Read the model definition and answer for the solid it produces. Units are mm, in the model's axes. Face numbers are marked on the shaded views. A direction names the side the tool comes from. Coordinates: 2 decimals unless noted, no trailing zeros. Order: outer loops, then holes, each group sorted by start corner. A loop starts at its lowest first (then second) coordinate and runs counter-clockwise, first axis right, second up. Notation, with made-up numbers: (-8, 61.5) -> (48, 61.5) arc R10 ccw to (48, 78.5) -> close; hole circle Ø4 at (75, 36.5). An arc over 180 degrees is marked (long way). Answer as a JSON object with one key per item and string values. Group by question number.
1) Section B-B on x = 12 is taken. Determine the outline of the cut face in (y, z), and give its area (3 significant figures).
2) Section D-D on x = -21 is taken. Determine the outline of the cut face in (y, z), and give its area (3 significant figures).
3) A tool of negligible diameter and unlimited length cuts with its end or side. For the marked faces 1, 2 and 3, from which of +Z, -Z, +X, -X, +Y, -Y can it reach the whole face along a straight path? Write none if from no direction.
4) Determine the mould class of the marked faces 4, 5 and 6 for opening direction Z: released by +Z, released by -Z, zero draft, split by the parting line, or undercut.
5) Consider L1, parallel to Z at x = -8.5, y = 28; L2, parallel to Z at x = -13.5, y = 20.5; L3, parallel to X at y = 20.5, z = 13. Determine where each line is inside the solid, lowest interval first.
6) Section A-A on y = 16.5 is taken. Determine the outline of the cut face in (x, z).
7) Given pin 1 (8 mm diameter, centred on x = 3, y = 17.5, fed in from +Z); pin 2 (8 mm diameter, centred on x = 26, y = 25, fed in from +Z); pin 3 (5 mm diameter, centred on y = 11.5, z = 112, fed in from +X); pin 4 (12 mm diameter, centred on x = 6.5, z = 48.5, fed in from +Y), each flat-ended and moving along its own axis, determine where each tip first touches the part or whether it passes through.
8) Section C-C on z = 24.5 is taken. Determine the outline of the cut face in (x, y).
from build123d import *

# Parameters (mm, degrees)
BOSS_EXTRUDE1_DEPTH = 30


with BuildPart() as part:
    # Sketch1 → Boss-Extrude1 (new body)
    with BuildSketch(Plane(origin=(0, 0, 0), x_dir=(1, 0, 0), z_dir=(0, 1, 0))):
        with BuildLine():
            Line((2, -107.749471884), (33.038610535, -107.749471884))
            Line((33.038610535, -107.749471884), (33.038610535, -103.749471884))
            Line((33.038610535, -103.749471884), (2, -103.749471884))
            Line((2, -103.749471884), (2, -35.811953605))
            Line((2, -35.811953605), (30.435409652, 0))
            Line((30.435409652, 0), (27.302817395, 2.487341101))
            Line((27.302817395, 2.487341101), (2, -29.379381894))
            Line((2, -29.379381894), (2, 0))
            Line((2, 0), (-2, 0))
            Line((-2, 0), (-2, -29.379381894))
            Line((-2, -29.379381894), (-27.302817395, 2.487341101))
            Line((-27.302817395, 2.487341101), (-30.435409652, 0))
            Line((-30.435409652, 0), (-2, -35.811953605))
            Line((-2, -35.811953605), (-2, -103.749471884))
            Line((-2, -103.749471884), (-33.038610535, -103.749471884))
            Line((-33.038610535, -103.749471884), (-33.038610535, -107.749471884))
            Line((-33.038610535, -107.749471884), (-2, -107.749471884))
            Line((-2, -107.749471884), (-2, -125.214231971))
            ThreePointArc((-2, -125.214231971), (0, -161.548956818), (2, -125.214231971))
            Line((2, -125.214231971), (2, -107.749471884))
        make_face()
    extrude(amount=BOSS_EXTRUDE1_DEPTH)


solid = part.part
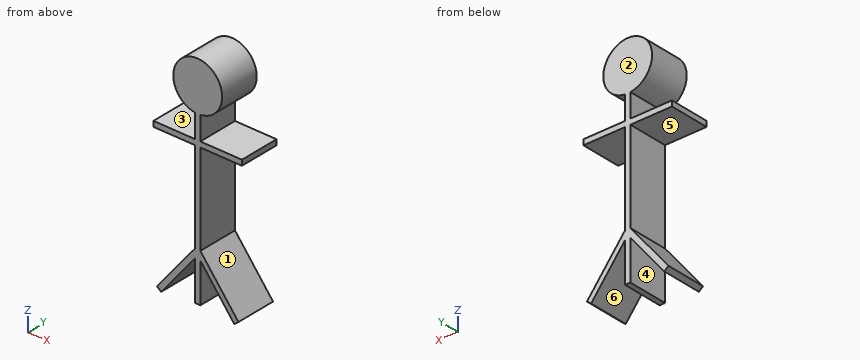
Worked answers:
{
 "1": {"outline": "(0, 16.79) -> (30, 16.79) -> (30, 23.22) -> (0, 23.22) -> close; (0, 103.75) -> (30, 103.75) -> (30, 107.75) -> (0, 107.75) -> close; (0, 129.61) -> (30, 129.61) -> (30, 157.04) -> (0, 157.04) -> close", "area": "1,140 mm²"},
 "2": {"outline": "(0, 5.45) -> (30, 5.45) -> (30, 11.88) -> (0, 11.88) -> close; (0, 103.75) -> (30, 103.75) -> (30, 107.75) -> (0, 107.75) -> close", "area": "313 mm²"},
 "3": {"face 1": "+X, +Y, -Y", "face 2": "+Z, -Z, +X, -X, +Y", "face 3": "-X, +Y, -Y"},
 "4": {"face 4": "zero draft", "face 5": "undercut", "face 6": "released by -Z"},
 "5": {"L1": "z = 21.19 to 27.63, 103.75 to 107.75, 127.21 to 159.45", "L2": "z = 14.9 to 21.33, 103.75 to 107.75, 131.09 to 155.57", "L3": "x = -20.11 to -15.01, -2 to 2, 15.01 to 20.11"},
 "6": {"outline": "(-33.04, 103.75) -> (-2, 103.75) -> (-2, 35.81) -> (-30.44, 0) -> (-27.3, -2.49) -> (-2, 29.38) -> (-2, 0) -> (2, 0) -> (2, 29.38) -> (27.3, -2.49) -> (30.44, 0) -> (2, 35.81) -> (2, 103.75) -> (33.04, 103.75) -> (33.04, 107.75) -> (2, 107.75) -> (2, 125.21) arc R18.22 ccw (long way) to (-2, 125.21) -> (-2, 107.75) -> (-33.04, 107.75) -> close"},
 "7": {"pin 1": "stops at z = 161.55", "pin 2": "stops at z = 107.75", "pin 3": "stops at x = 2", "pin 4": "stops at y = 30"},
 "8": {"outline": "(-10.98, 0) -> (-5.87, 0) -> (-5.87, 30) -> (-10.98, 30) -> close; (-2, 0) -> (2, 0) -> (2, 30) -> (-2, 30) -> close; (5.87, 0) -> (10.98, 0) -> (10.98, 30) -> (5.87, 30) -> close"}
}
